Could you check a few things on this model? Use its own coordinates, in mm. A direction names the side the tool comes from. Give positions to 0.01 mm unless a question says otherwise; leave off trailing zeros. Loops run counter-clockwise (first coordinate to the right, second up) from the corner with the lowest first, then second, coordinate; pieces in that order, holes last. Notation, with made-up numbers: (51, 14.25) -> (67, 14.25) arc R29 ccw to (67, 41.25) -> close; hole circle Ø2 at (34, -30). An arc over 180 degrees is marked (long way). Write each question's results on one line, items separated by ' | '. Start each with the question number.
Q1. If we section it at D-D, the plane x = 173.5: List the corners of the cut face in (y, z) for me, plus the area to 3 significant figures.
Q2. If we section it at A-A, the plane z = 0: List the corners of the cut face in (x, y) for me, plus the area to 3 significant figures.
Q3. Which directions (+Z, -Z, +X, -X, +Y, -Y) give clear straight access to the entire face, cutting with the end or side of a thin tool? Please do faces 5 (the face through (35.311, -10.548, 33.494)), 6 (the face through (171.806, 22.534, 11.721)), 7 (the face through (0, -17, 31)).
Q4. If I drill on line 1 along Y through (x, z) = (38.5, 0); line 2 along Y through (x, z) = (178.5, 0); line 3 along Z through (x, y) = (120, -22.5), over which ranges is the centre line in solid material (lowest first)?
Q5. We'd pull the mould along Z, two halves only. Please class faces 1 (the face through (196.85, -10, -21)), 2 (the face through (171.71, 13.91, -18.14)), 3 (the face through (116.75, 24.43, 12.71)), 4 (the face through (35.41, 36.76, -8.16)): released by +Z, released by -Z, zero draft, split by the parting line, or undercut.
Q6. If we section it at C-C, the plane x = 21: List the corners of the cut face in (y, z) for me, plus the area to 3 significant figures.
Q7. Will these pins go through, and if not, where does the flat tip stop? P1, Ø4, axis at x = 88, y = -10.5, coming from the -Z side; P2, Ø4, axis at x = 90.5, y = 20.5, coming from the -Z side; P3, Ø4, axis at x = 53, z = 17, coming from the +Y side.
from build123d import *

# Parameters (mm, degrees)
SHELL1_T = -2.54


with BuildPart() as part:
    # Sketch1 → Revolve1 (revolve)
    with BuildSketch(Plane(origin=(0, 0, 0), x_dir=(1, 0, 0), z_dir=(0, 1, 0)), mode=Mode.PRIVATE) as revolve1_sk:
        Polygon((0, 0), (0, 37.6555), (69.85, 37.6555), (146.05, 25.4), (196.85, 25.4), (196.85, 0), align=None)
    revolve(revolve1_sk.sketch.rotate(Axis((0, 0, 0), (1, 0, 0)), 180), axis=Axis((0, 0, 0), (1, 0, 0)))

    # Shell1
    shell1_openings = [part.faces().sort_by_distance(p)[0] for p in [
        (196.85, 0, 0),
        (0, 0, 0),
    ]]
    offset(amount=SHELL1_T, openings=shell1_openings, kind=Kind.INTERSECTION)


solid = part.part
Final values:
1) outline: circle Ø50.8 at (0, 0); hole circle Ø45.72 at (0, 0) | area: 385 mm²
2) outline: (0, -37.66) -> (69.85, -37.66) -> (146.05, -25.4) -> (196.85, -25.4) -> (196.85, -22.86) -> (145.85, -22.86) -> (69.65, -35.12) -> (0, -35.12) -> close; (0, 35.12) -> (69.65, 35.12) -> (145.85, 22.86) -> (196.85, 22.86) -> (196.85, 25.4) -> (146.05, 25.4) -> (69.85, 37.66) -> (0, 37.66) -> close | area: 1,000 mm²
3) face 5: -X | face 6: +X | face 7: +Z, -Z, -X, +Y, -Y
4) line 1: y = -37.66 to -35.12, 35.12 to 37.66 | line 2: y = -25.4 to -22.86, 22.86 to 25.4 | line 3: z = -19.22 to -14.96, 14.96 to 19.22
5) face 1: zero draft | face 2: undercut | face 3: undercut | face 4: split by the parting line
6) outline: circle Ø75.31 at (0, 0); hole circle Ø70.23 at (0, 0) | area: 581 mm²
7) P1: stops at z = -33.78 | P2: stops at z = -28.98 | P3: stops at y = 34.54
